Verification items for this drawing (mm, ordinates from the low corner). Coordinates: 2 decimals unless noted, no trailing zeros. Order: outer loops, then holes, each group sorted by start corner. A loop starts at its lowest first (then second) coordinate and runs counter-clockwise, first axis right, second up.
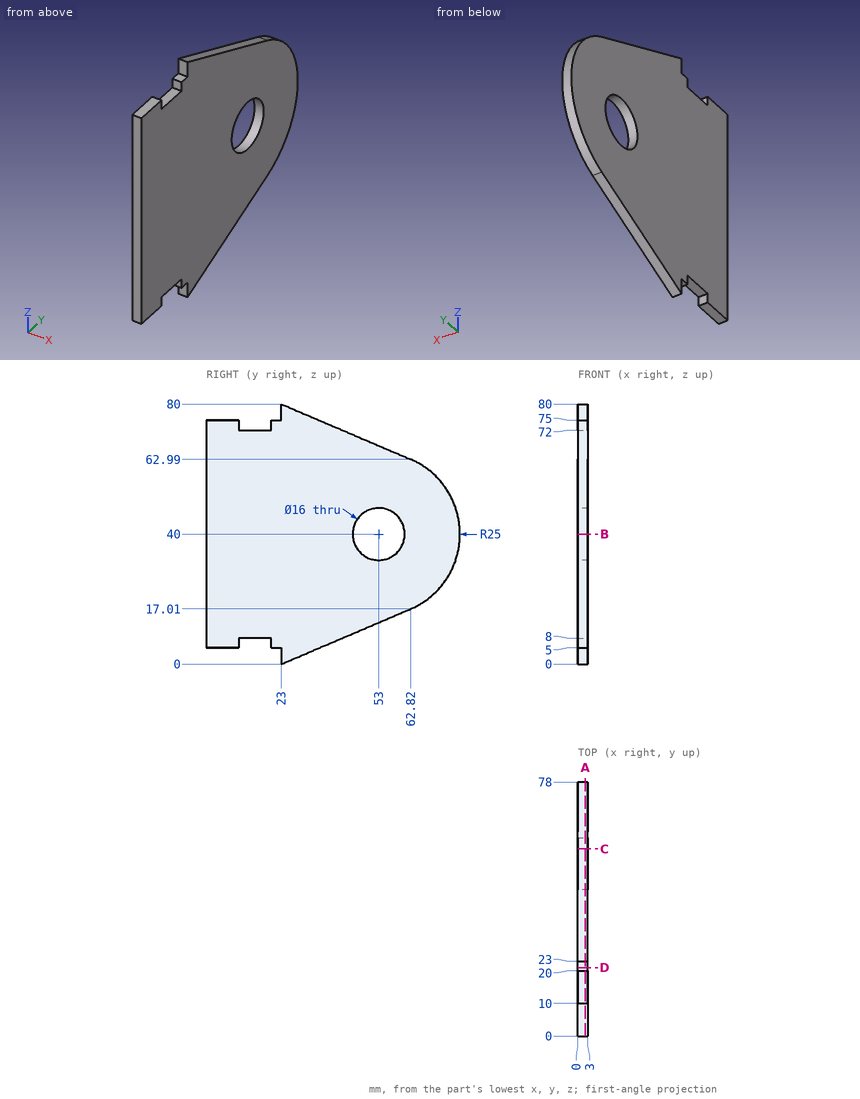
(1) Cross-section at C-C (y = 57.5). Enter the section's corners in (x, z) (1 decimal), and give its area (3 significant figures).
Filled in:
outline: (0, 14.7) - (3, 14.7) - (3, 33.4) - (0, 33.4) - close; (0, 46.6) - (3, 46.6) - (3, 65.3) - (0, 65.3) - close
area: 112 mm2
(2) Cross-section at A-A (x = 2.25). Enter the section's corners in (y, z).
Filled in:
outline: (0, 5) - (10, 5) - (10, 8) - (20, 8) - (20, 5) - (23, 5) - (23, 0) - (62.82, 17.01) arc R25 ccw to (62.82, 62.99) - (23, 80) - (23, 75) - (20, 75) - (20, 72) - (10, 72) - (10, 75) - (0, 75) - close; hole circle Ø16 at (53, 40)
(3) Cross-section at D-D (y = 21). Enter the section's corners in (x, z).
Filled in:
outline: (0, 5) - (3, 5) - (3, 75) - (0, 75) - close
(4) Thickness scan on probe 1 along Z at (x, y) = (2.15, 16); probe 2 along Z at (x, y) = (2, 53) (1 decimal); probe 3 along Z at (x, y) = (0.8, 59) (1 decimal). Record the ranges inside material, lowest first.
Filled in:
probe 1: z = 8 to 72
probe 2: z = 12.8 to 32, 48 to 67.2
probe 3: z = 15.4 to 34.7, 45.3 to 64.6
(5) Go/stop test with flat-tipped pins: P1, Ø1.5, axis at x = 1, z = 10.5, coming from the +Y side (1 decimal); P2, Ø1.5, axis at x = 1.5, z = 2.5, coming from the -Y side; P3, Ø0.9, axis at x = 1, z = 7, coming from the +Y side. Record where each tip stops, or that it passes through.
Filled in:
P1: stops at y = 49.3
P2: stops at y = 23
P3: stops at y = 40.44
(6) Cross-section at B-B (z = 40). Enter the section's corners in (x, y).
Filled in:
outline: (0, 0) - (3, 0) - (3, 45) - (0, 45) - close; (0, 61) - (3, 61) - (3, 78) - (0, 78) - close
